The drawing under review shows one solid part. Ordinate dimensions are in mm from its lowest x, y, z. A direction names the side the tool comes from. Round coordinates to 2 decimals unless told otherwise and drop trailing zeros. Order: outer loops, then holes, each group sorted by start corner. A loop starts at its lowest first (then second) coordinate and runs counter-clockwise, first axis right, second up. Notation, with made-up numbers: (55.25, -6.75) - (70.25, -6.75) arc R21 ccw to (70.25, 4.25) - close; hole circle Ø2 at (62, 2). An arc over 180 degrees is marked (long way). One line per question, with ' | ' between items.
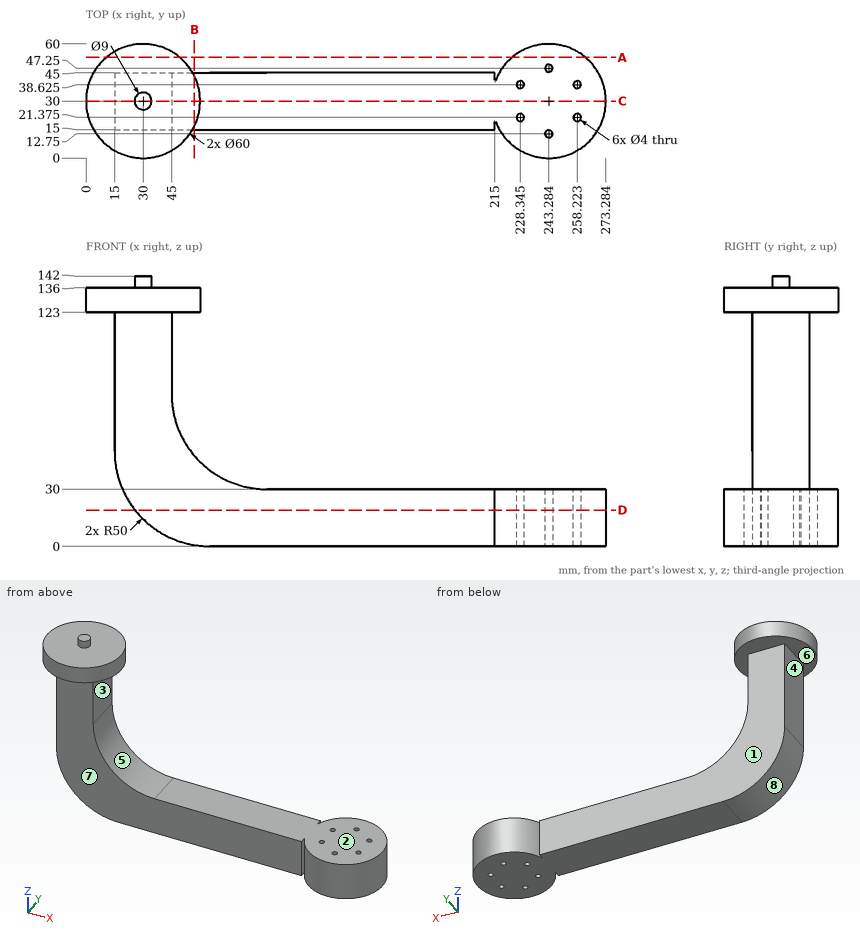
(1) We need section D-D on z = 19. Give the number of separate pieces and of enclosed holes in the cut face, plus the area to 3 significant figures.
Output values:
separate pieces: 1 | enclosed holes: 6 | area: 8,410 mm^2
(2) We need section A-A on y = 53. State the section outline as (x, z) points (1 decimal).
Output values:
outline: (10.7, 123) - (49.3, 123) - (49.3, 136) - (10.7, 136) - close; (224, 0) - (262.5, 0) - (262.5, 30) - (224, 30) - close
(3) For the marked faces 1, 2, 3 and 4, list the 3-axis set-ups (+Z, -Z, +X, -X, +Y, -Y) from which the entire face can be reached by the end or side of a thin tool; tool diameter is ignored.
Output values:
face 1: -Z, -X, +Y | face 2: +Z, +X, +Y, -Y | face 3: +X, +Y, -Y | face 4: -Z, -X, +Y, -Y
(4) We need section C-C on y = 30. State the section outline as (x, z) points.
Output values:
outline: (0, 123) - (15, 123) - (15, 50) arc R50 ccw to (65, 0) - (273.28, 0) - (273.28, 30) - (95, 30) arc R50 cw to (45, 80) - (45, 123) - (60, 123) - (60, 136) - (34.5, 136) - (34.5, 142) - (25.5, 142) - (25.5, 136) - (0, 136) - close
(5) We need section B-B on x = 57. State the section outline as (y, z) points, plus the area to 3 significant figures.
Output values:
outline: (15, 0.64) - (45, 0.64) - (45, 47.5) - (15, 47.5) - close; (16.92, 123) - (43.08, 123) - (43.08, 136) - (16.92, 136) - close | area: 1,750 mm^2
(6) Mouldability with a two-part tool opening along Z and no side actions: class the marked faces 5, 6, 7 and 8 as released by +Z, released by -Z, zero draft, split by the parting line, or undercut.
Output values:
face 5: undercut | face 6: undercut | face 7: zero draft | face 8: released by -Z
(7) For probe 1 along Z at (x, y) = (156, 15.5); probe 2 along Y at (x, z) = (37, 67); probe 3 along X at (y, z) = (18, 10.5) (1 decimal), list the stretches that pass through material, from the lowest coordinate up. Write a range as [from, to].
Output values:
probe 1: [0, 30] | probe 2: [15, 45] | probe 3: [34.3, 215], [215.8, 270.8]
(8) Insertion check: pin 1 (5 mm diameter, centred on x = 121, z = 21.5, fed in from -Y); pin 2 (9 mm diameter, centred on y = 37, z = 76.5, fed in from -X); pin 3 (3 mm diameter, centred on x = 228.35, y = 38.62, fed in from +Z); pin 4 (1 mm diameter, centred on x = 229.5, z = 23.5, fed in from +Y). Each pin has a flat end and moves straight along its axis. Give the tip position at first contact, or say it passes through.
Output values:
pin 1: y = 15 | pin 2: x = 15 | pin 3: through | pin 4: y = 56.9
